Part model, mm, in its own coordinate system. Face numbers are marked on the shaded views. A direction names the side the tool comes from. Round coordinates to 2 decimals unless told otherwise and drop trailing zeros. Loops run counter-clockwise (first coordinate to the right, second up) from the corner with the lowest first, then second, coordinate; pieces in that order, holes last. Notation, with made-up numbers: (13.5, 37.25) - (69.5, 37.25) arc R21 cw to (69.5, 53.25) - close; hole circle Ø4 at (-5.5, 89.25). An arc over 180 degrees is marked (long way). Write each question's results on one line, items separated by ' | '. Start each with the question number.
(1) Cut at C-C, the plane z = 6.5. List the corners of the cut face in (x, y), then the cut area to 3 significant figures.
(2) Cut at A-A, the plane z = 31. List the corners of the cut face in (x, y).
(3) Flat gauge pins, fed straight in: P1, Ø5, axis at x = -106.03, y = 24.69, coming from the +Z side; P2, Ø10, axis at x = -70.5, z = 37.5, coming from the +Y side; P3, Ø4, axis at x = -85.5, z = 9.5, coming from the -Y side. Where does each tip first touch, or does it go through?
(4) Mould opens along X. For the marked faces 1, 2, 3 and 4 say: released by +X, released by -X, zero draft, split by the parting line, or undercut.
(5) Tool access for the marked faces 5, 6, 7 and 8: list every direction of +Z, -Z, +X, -X, +Y, -Y with a clear straight run to the whole face (end or side of a thin tool).
(6) Cut at B-B, the plane y = 39. List the corners of the cut face in (x, z), then the cut area to 3 significant figures.
(7) Cut at D-D, the plane y = 45.25. List the corners of the cut face in (x, z).
(8) Drill centre lines: L1, parallel to Y at x = -97.5, z = 26.5; L2, parallel to Z at x = -109.5, y = 21.5; L3, parallel to Z at x = -106.5, y = 30.5. Where is each one in solid material? Low to high.
from build123d import *

# Parameters (mm, degrees)
SKETCH1_W           = 60
SKETCH1_H           = 4
BOSS_EXTRUDE1_DEPTH = 45
SKETCH1_3_R         = 2.2
BOSS_EXTRUDE2_DEPTH = 5
SKETCH2_R           = 3
SKETCH2_R_2         = 1.6
CUT_EXTRUDE1_DEPTH  = 5
BOSS_EXTRUDE3_DEPTH = 45
FILLET1_R           = 2.5
FILLET3_R           = 2.5
SKETCH3_R           = 4
BOSS_EXTRUDE4_DEPTH = 13
SKETCH4_R           = 6
BOSS_EXTRUDE5_DEPTH = 5
FILLET4_R           = 1
SKETCH6_W           = 45
SKETCH6_H           = 16
CUT_EXTRUDE2_DEPTH  = 61


with BuildPart() as part:
    # Sketch1 → Boss-Extrude1 (new body)
    with BuildSketch(Plane.XY):
        with Locations((-82.025641026, 5.685176195)):
            Rectangle(SKETCH1_W, SKETCH1_H)
    extrude(amount=BOSS_EXTRUDE1_DEPTH)

    # Sketch1_3 → Boss-Extrude2 (add)
    with BuildSketch(Plane.XY):
        Polygon((-112.025641026, 27.185176195), (-112.025641026, 7.685176195), (-103.025641026, 7.685176195), (-103.025641026, 27.185176195), (-103.025641026, 31.685176195), (-112.025641026, 31.685176195), align=None)
        with Locations((-106.025641026, 14.685176195)):
            Circle(SKETCH1_3_R, mode=Mode.SUBTRACT)
        with Locations((-106.025641026, 24.685176195)):
            Circle(SKETCH1_3_R, mode=Mode.SUBTRACT)
        Polygon((-61.025641026, 27.185176195), (-61.025641026, 7.685176195), (-52.025641026, 7.685176195), (-52.025641026, 27.185176195), (-52.025641026, 31.685176195), (-61.025641026, 31.685176195), align=None)
        with Locations((-58.025641026, 14.685176195)):
            Circle(SKETCH1_3_R, mode=Mode.SUBTRACT)
        with Locations((-58.025641026, 24.685176195)):
            Circle(SKETCH1_3_R, mode=Mode.SUBTRACT)
    extrude(amount=BOSS_EXTRUDE2_DEPTH)

    # Sketch2 → Cut-Extrude1 (cut, through all)
    with BuildSketch(Plane(origin=(0, 7.685176195, 0), x_dir=(1, 0, 0), z_dir=(0, 1, 0))):
        with Locations((-82.025641026, -31)):
            Circle(SKETCH2_R)
        with Locations((-77.025641026, -26)):
            Circle(SKETCH2_R_2)
        with Locations((-87.025641026, -26)):
            Circle(SKETCH2_R_2)
        with Locations((-77.025641026, -36)):
            Circle(SKETCH2_R_2)
        with Locations((-87.025641026, -36)):
            Circle(SKETCH2_R_2)
    extrude(amount=-CUT_EXTRUDE1_DEPTH, mode=Mode.SUBTRACT)

    # Sketch1_4 → Boss-Extrude3 (add)
    with BuildSketch(Plane.XY):
        Polygon((-112.025641026, 35.685176195), (-112.025641026, 31.685176195), (-103.025641026, 31.685176195), (-61.025641026, 31.685176195), (-52.025641026, 31.685176195), (-52.025641026, 35.685176195), align=None)
    extrude(amount=BOSS_EXTRUDE3_DEPTH)

    # Fillet1
    fillet1_edges = [part.edges().sort_by_distance(p)[0] for p in [
        (-112.025641026, 5.685176195, 45),
        (-52.025641026, 5.685176195, 45),
        (-112.025641026, 33.685176195, 45),
        (-52.025641026, 33.685176195, 45),
    ]]
    fillet(fillet1_edges, radius=FILLET1_R)

    # Fillet3
    fillet3_edges = [part.edges().sort_by_distance(p)[0] for p in [
        (-107.525641026, 31.685176195, 5),
        (-107.525641026, 7.685176195, 5),
        (-56.525641026, 31.685176195, 5),
        (-56.525641026, 7.685176195, 5),
    ]]
    fillet(fillet3_edges, radius=FILLET3_R)

    # Sketch3 → Boss-Extrude4 (add)
    with BuildSketch(Plane(origin=(0, 35.685176195, 0), x_dir=(1, 0, 0), z_dir=(0, 1, 0))):
        with Locations((-82.025641026, -31)):
            Circle(SKETCH3_R)
    extrude(amount=BOSS_EXTRUDE4_DEPTH)

    # Sketch4 → Boss-Extrude5 (add)
    with BuildSketch(Plane(origin=(0, 35.685176195, 0), x_dir=(1, 0, 0), z_dir=(0, 1, 0))):
        with Locations((-82.025641026, -31)):
            Circle(SKETCH4_R)
    extrude(amount=BOSS_EXTRUDE5_DEPTH)

    # Fillet4
    fillet4_edges = [part.edges().sort_by_distance(p)[0] for p in [
        (-86.025641026, 40.685176195, 31),
    ]]
    fillet(fillet4_edges, radius=FILLET4_R)

    # Sketch6 → Cut-Extrude2 (cut, through all)
    with BuildSketch(Plane(origin=(-52.025641026, 0, 0), x_dir=(0, 0, -1), z_dir=(1, 0, 0))):
        with Locations((-22.5, 11.685176195)):
            Rectangle(SKETCH6_W, SKETCH6_H)
    extrude(amount=-CUT_EXTRUDE2_DEPTH, mode=Mode.SUBTRACT)


solid = part.part
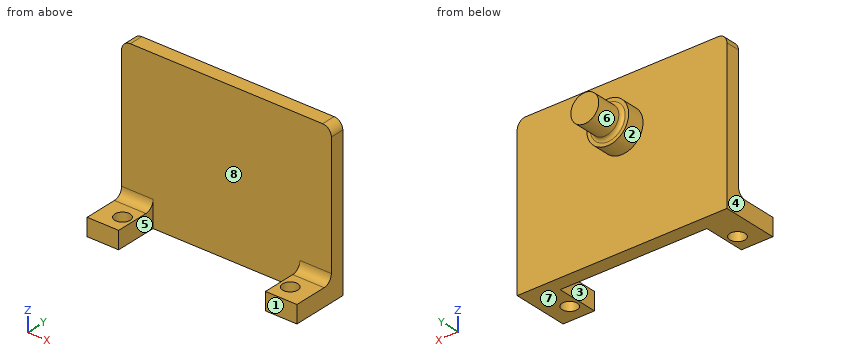
A:
1) outline: (-112.03, 31.48) - (-103.03, 31.48) - (-103.03, 31.69) - (-61.03, 31.69) - (-61.03, 31.48) - (-52.03, 31.48) - (-52.03, 35.69) - (-112.03, 35.69) - close | area: 244 mm2
2) outline: (-112.03, 31.69) - (-52.03, 31.69) - (-52.03, 35.69) - (-76.03, 35.69) - (-76.03, 40.69) - (-77.03, 40.69) arc R1 cw to (-78.03, 41.69) - (-78.03, 48.69) - (-86.03, 48.69) - (-86.03, 41.69) arc R1 cw to (-87.03, 40.69) - (-88.03, 40.69) - (-88.03, 35.69) - (-112.03, 35.69) - close
3) P1: z = 5 | P2: y = 35.69 | P3: y = 31.69
4) face 1: zero draft | face 2: split by the parting line | face 3: undercut | face 4: released by -X
5) face 5: +Z, -Z, -Y | face 6: +Y | face 7: -Z, +X, -X, +Y, -Y | face 8: +Z, -Y
6) outline: circle Ø12 at (-82.03, 31) | area: 113 mm2
7) outline: circle Ø8 at (-82.03, 31)
8) L1: 31.69 to 35.69 | L2: 0 to 5 | L3: 0 to 5.37
